Here's how the part is built. I have some questions about the finished solid (model axes, mm). Coordinates: 2 decimals unless noted, no trailing zeros. Order: outer loops, then holes, each group sorted by start corner. A loop starts at its lowest first (then second) coordinate and runs counter-clockwise, first axis right, second up. Notation, with made-up numbers: (55, 73.5) - (80, 73.5) arc R26 ccw to (80, 95.5) - close; hole circle Ø2 at (7, -21). An arc over 180 degrees is marked (long way). Answer in a Markdown table with one row per item. Add a question column.
Item 1: I want a section at D-D (x = 12). Please give me the cut outline in (y, z).
Item 2: Thinking about a two-plate mould opening in X: for faces 1 (the cylindrical face through (11.54, 0.99, -26.12)), 2 (the cylindrical face through (-30.5, 1, 12.6)), 3 (the flat face through (-7, 0, -7)), 4 (the cylindrical face through (1.73, 0.99, 7.81)), which applies, +X half, -X half, draft (parallel to the pull), parting line (faces both ways), or undercut?
Item 3: I want a section at C-C (z = -19.5). Please give me the cut outline in (x, y).
Item 4: If I drill on line 1 along X through (y, z) = (1.15, 24); line 2 along Z through (x, y) = (-4, 0.1); line 3 along X through (y, z) = (1.35, -7), over which ranges is the centre line in solid material (lowest first)? Write a range as from..to.
Item 5: I want a section at B-B (z = 1.5). Please give me the cut outline in (x, y), plus the area to 3 significant figures.
Item 6: I want a section at A-A (x = 0). Please give me the cut outline in (y, z).
Autodesk Inventor part; units mm, degrees
ref_plane "YZ Plane" through (0, 0, 0) normal (1, 0, 0) x (0, 1, 0)
ref_plane "XZ Plane" through (0, 0, 0) normal (0, 1, 0) x (-1, 0, 0)
ref_plane "XY Plane" through (0, 0, 0) normal (0, 0, 1) x (1, 0, 0)
sketch "Sketch3" plane through (0, 0, 0) normal (0, 1, 0) x (-1, 0, 0)
  circle A0 centre (0, 0) radius 33
  circle A1 centre (0, 0) radius 8
  line L0 (0, 0) -> (32, 0) construction
  line L1 (0, 0) -> (34, 0) construction
  line L2 (24.0416, -24.0416) -> (20.5061, -20.5061)
  line L3 (0, 0) -> (34, 0) construction
  line L4 (0, 0) -> (22.2739, 0)
  line L5 (0, 0) -> (21, 0)
  circle A2 centre (21, 0) radius 8
  circle A3 centre (10.5, 18.1865) radius 8
  circle A4 centre (-10.5, 18.1865) radius 8
  circle A5 centre (-21, 0) radius 8
  circle A6 centre (-10.5, -18.1865) radius 8
  circle A7 centre (10.5, -18.1865) radius 8
  dimension "d15" = 66
  dimension "d17" = 16
  dimension "d25" = 34
  dimension "d27" = 5
  dimension "d31" = 21
  dimension "d32" = 16
  dimension "d35" = 360
extrude "Extrusion1" add sketch "Sketch3" along normal blind 2
properties part number "separator"
Values follow:
| question | item | result |
|---|---|---|
| 1 | outline | (0, -30.74) - (2, -30.74) - (2, -26.04) - (0, -26.04) - close; (0, -10.33) - (2, -10.33) - (2, 10.33) - (0, 10.33) - close; (0, 26.04) - (2, 26.04) - (2, 30.74) - (0, 30.74) - close |
| 2 | face 1 | undercut |
| 2 | face 2 | parting line |
| 2 | face 3 | draft |
| 2 | face 4 | undercut |
| 3 | outline | (-26.62, 0) - (-18.39, 0) - (-18.39, 2) - (-26.62, 2) - close; (-2.61, 0) - (2.61, 0) - (2.61, 2) - (-2.61, 2) - close; (18.39, 0) - (26.62, 0) - (26.62, 2) - (18.39, 2) - close |
| 4 | line 1 | x = -22.65..-16, -5..5, 16..22.65 |
| 4 | line 2 | z = -32.76..-22.85, -13.52..-6.93, 6.93..13.52, 22.85..32.76 |
| 4 | line 3 | x = -32.25..-24.87, -17.13..-3.87, 3.87..17.13, 24.87..32.25 |
| 5 | outline | (-32.97, 0) - (-28.86, 0) - (-28.86, 2) - (-32.97, 2) - close; (-13.14, 0) - (-7.86, 0) - (-7.86, 2) - (-13.14, 2) - close; (7.86, 0) - (13.14, 0) - (13.14, 2) - (7.86, 2) - close; (28.86, 0) - (32.97, 0) - (32.97, 2) - (28.86, 2) - close |
| 5 | area | 37.6 mm^2 |
| 6 | outline | (0, -33) - (2, -33) - (2, -8) - (0, -8) - close; (0, 8) - (2, 8) - (2, 33) - (0, 33) - close |
